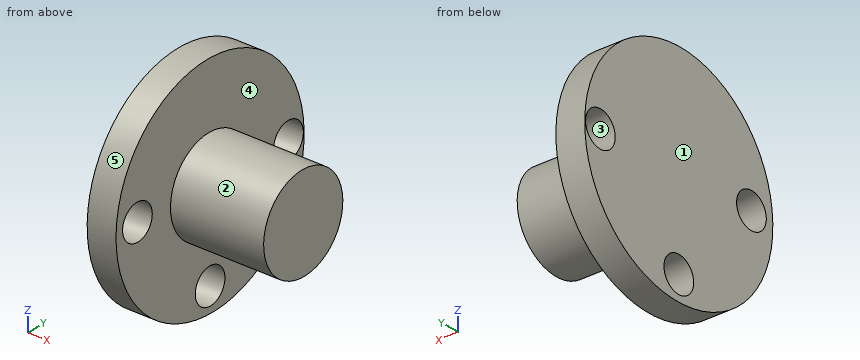
from build123d import *

# Parameters (mm, degrees)
F2_R     = 9.525
F3_DEPTH = 508.508
F4_R     = 9.525
F5_DEPTH = 25.4
F6_R     = 9.525
F7_DEPTH = 25.4


with BuildPart() as f1:
    # F0 (on Front) → F1 (revolve)
    with BuildSketch(Plane.XZ):
        Polygon((-45.004993, 53.025745), (-60.752993, 53.025745), (-60.752993, -7.299255), (5.795007, -7.299255), (5.795007, 18.100745), (-45.004993, 18.100745), align=None)
    revolve(axis=Axis((-27.478993, 0, -7.299255), (1, 0, 0)))

    # F2 (on face) → F3 (cut)
    with BuildSketch(Plane.YZ.offset(-45.004993)):
        with Locations((50.308675, -6.467566)):
            Circle(F2_R)
    extrude(amount=-F3_DEPTH, mode=Mode.SUBTRACT)

    # F4 (on face) → F5 (cut)
    with BuildSketch(Plane.YZ.offset(-45.004993)):
        with Locations((-46.595834, -5.428873)):
            Circle(F4_R)
    extrude(amount=-F5_DEPTH, mode=Mode.SUBTRACT)

    # F6 (on face) → F7 (cut)
    with BuildSketch(Plane.YZ.offset(-45.004993)):
        with Locations((0, -54.508783)):
            Circle(F6_R)
    extrude(amount=-F7_DEPTH, mode=Mode.SUBTRACT)


solid = f1.part
Build history of the part. All positions in model axes, mm. Face numbers are marked on the shaded views. A direction names the side the tool comes from. Give positions to 0.01 mm unless a question says otherwise; leave off trailing zeros. Loops run counter-clockwise (first coordinate to the right, second up) from the corner with the lowest first, then second, coordinate; pieces in that order, holes last. Notation, with made-up numbers: (5, -5) -> (49, -5) arc R27 ccw to (49, 28) -> close; hole circle Ø3 at (3.5, 48.25). An arc over 180 degrees is marked (long way). Answer in a Markdown table with one row per item.
Item 1: Probe line 1 along X through (y, z) = (-1, 27.5) (3 decimals); line 2 along Z through (x, y) = (-57.5, 0); line 3 along Z through (x, y) = (-2, 1). List the from-to ranges inside material, lowest first. Write a range as [from, to].
Findings below:
| item | result |
|---|---|
| line 1 | x = [-60.753, -45.005] |
| line 2 | z = [-67.62, -64.03], [-44.98, 53.03] |
| line 3 | z = [-32.68, 18.08] |
Item 2: Flat gauge pins, fed straight in: P1, Ø4, axis at x = -20, y = -20.5, coming from the +Z side; P2, Ø5, axis at x = -1.5, z = -11, coming from the +Y side; P3, Ø17, axis at y = 0, z = -54.51, coming from the +X side; P4, Ø6, axis at x = -24.5, y = 12, coming from the -Z side. Where does each tip first touch, or does it go through?
Findings below:
| item | result |
|---|---|
| P1 | stops at z = 10.11 |
| P2 | stops at y = 25.37 |
| P3 | passes through |
| P4 | stops at z = -31.05 |
Item 3: Slice it at C-C on z = 7.5. Write the cut outline in (x, y) (3 decimals).
Findings below:
| item | result |
|---|---|
| outline | (-60.753, -58.482) -> (-45.005, -58.482) -> (-45.005, -20.643) -> (5.795, -20.643) -> (5.795, 20.643) -> (-45.005, 20.643) -> (-45.005, 58.482) -> (-60.753, 58.482) -> close |
Item 4: Mould opens along Y. For the marked faces 1, 2 and 3 say: pulls with the +Y half, pulls with the -Y half, needs draft (parallel to the pull), parting line crosses it, or undercut.
Findings below:
| item | result |
|---|---|
| face 1 | needs draft |
| face 2 | parting line crosses it |
| face 3 | undercut |
Item 5: Slice it at B-B on z = -47.5. Write the cut outline in (x, y) (3 decimals).
Findings below:
| item | result |
|---|---|
| outline | (-60.753, -44.978) -> (-45.005, -44.978) -> (-45.005, -6.45) -> (-60.753, -6.45) -> close; (-60.753, 6.45) -> (-45.005, 6.45) -> (-45.005, 44.978) -> (-60.753, 44.978) -> close |
Item 6: Slice it at A-A on y = 0. Write the cut outline in (x, z) (3 decimals).
Findings below:
| item | result |
|---|---|
| outline | (-60.753, -67.624) -> (-45.005, -67.624) -> (-45.005, -64.034) -> (-60.753, -64.034) -> close; (-60.753, -44.984) -> (-45.005, -44.984) -> (-45.005, -32.699) -> (5.795, -32.699) -> (5.795, 18.101) -> (-45.005, 18.101) -> (-45.005, 53.026) -> (-60.753, 53.026) -> close |
Item 7: Tool access for the marked faces 4 and 5: list every direction of +Z, -Z, +X, -X, +Y, -Y with a clear straight run to the whole face (end or side of a thin tool).
Findings below:
| item | result |
|---|---|
| face 4 | +X |
| face 5 | +X, -X |
Item 8: Slice it at D-D on x = -51.5. Write the cut outline in (y, z) (3 decimals), plus the area to 3 significant figures.
Findings below:
| item | result |
|---|---|
| outline | circle Ø120.65 at (0, -7.299); hole circle Ø19.05 at (-46.596, -5.429); hole circle Ø19.05 at (0, -54.509); hole circle Ø19.05 at (50.309, -6.468) |
| area | 10,600 mm² |
